Here's the drawing with two shaded views (mm, measured from the low corner). I have some questions. A direction names the side the tool comes from. Coordinates: 2 decimals unless noted, no trailing zeros. Loops run counter-clockwise (first coordinate to the right, second up) from the corner with the lowest first, then second, coordinate; pieces in that order, holes last. Notation, with made-up numbers: (39, 69.5) - (93, 69.5) arc R23 cw to (93, 85.5) - close; hole circle Ø8 at (19, 33.5). An arc over 180 degrees is marked (long way). Use a Markdown table: item, result.
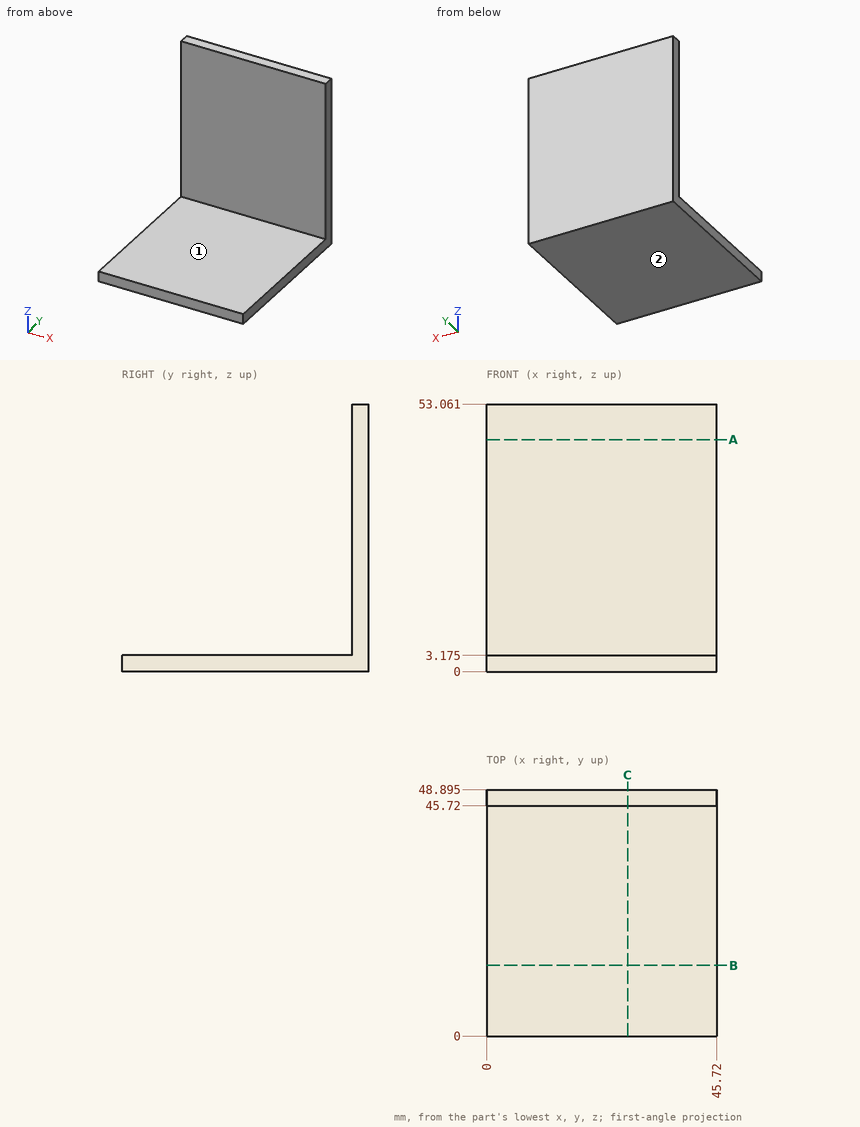
Q1. I want a section at A-A, the plane z = 46. Write out the boundary of the cut face in (x, y) (3 decimals), then the cut area to 3 significant figures.
Check values:
| item | result |
|---|---|
| outline | (0, 45.72) - (45.72, 45.72) - (45.72, 48.895) - (0, 48.895) - close |
| area | 145 mm^2 |
Q2. Which directions (+Z, -Z, +X, -X, +Y, -Y) give clear straight access to the entire face, cutting with the end or side of a thin tool? Please do the marked faces 1 and 2.
Check values:
| item | result |
|---|---|
| face 1 | +Z, +X, -X, -Y |
| face 2 | -Z, +X, -X, +Y, -Y |
Q3. Please list where these lines run through material, in increasing order: L1, parallel to Z at x = 16.5, y = 31.5 (3 decimals); L2, parallel to Y at x = 28, z = 17.5 (3 decimals). Write a range as from..to.
Check values:
| item | result |
|---|---|
| L1 | 0..3.175 |
| L2 | 45.72..48.895 |
Q4. Will these pins go through, and if not, where does the flat tip stop? P1, Ø4, axis at x = 24, z = 8.5, coming from the -Y side; P2, Ø23, axis at x = 34, y = 12.5, coming from the +Z side (3 decimals).
Check values:
| item | result |
|---|---|
| P1 | y = 45.72 |
| P2 | z = 3.175 |
Q5. I want a section at C-C, the plane x = 28. Write out the boundary of the cut face in (y, z) (1 decimal).
Check values:
| item | result |
|---|---|
| outline | (0, 0) - (48.9, 0) - (48.9, 53.1) - (45.7, 53.1) - (45.7, 3.2) - (0, 3.2) - close |
Q6. I want a section at B-B, the plane y = 14. Write out the boundary of the cut face in (x, z) (3 decimals), then the cut area to 3 significant figures.
Check values:
| item | result |
|---|---|
| outline | (0, 0) - (45.72, 0) - (45.72, 3.175) - (0, 3.175) - close |
| area | 145 mm^2 |
